Verification items for the finished model (mm, model axes). Give positions to 0.01 mm unless a question says otherwise; leave off trailing zeros. Write each loop counter-clockwise with the first axis right and the second up, starting at its lowest first coordinate (ties: lowest second). Pieces come first, ordered by that corner, then holes. Notation, with made-up numbers: (1, 68) -> (56, 68) arc R25 ccw to (56, 98) -> close; hole circle Ø5 at (3.5, -26.5). An arc over 180 degrees is marked (long way). Write item = value, one per line.
from build123d import *

# Parameters (mm, degrees)
SKETCH1_R           = 12.5
SKETCH1_R_2         = 1.5
SKETCH1_R_3         = 6
SKETCH1_R_4         = 4
BOSS_EXTRUDE1_DEPTH = 3
BOSS_EXTRUDE2_START = 3
SKETCH1_3_R         = 6
SKETCH1_3_R_2       = 4
BOSS_EXTRUDE2_DEPTH = 10


with BuildPart() as part:
    # Sketch1 → Boss-Extrude1 (new body)
    # profile 1 of 2: a face of its own
    with BuildSketch(Plane(origin=(0, 0, 0), x_dir=(1, 0, 0), z_dir=(0, 1, 0))):
        with Locations(Location((0, 0, 0), (0, 0, 270))):
            Circle(SKETCH1_R)
        with Locations(Location((-10, 0, 0), (0, 0, 270))):
            Circle(SKETCH1_R_2, mode=Mode.SUBTRACT)
        with Locations(Location((0, -10, 0), (0, 0, 270))):
            Circle(SKETCH1_R_2, mode=Mode.SUBTRACT)
        with Locations(Location((10, 0, 0), (0, 0, 270))):
            Circle(SKETCH1_R_2, mode=Mode.SUBTRACT)
        with Locations(Location((0, 10, 0), (0, 0, 270))):
            Circle(SKETCH1_R_2, mode=Mode.SUBTRACT)
        Circle(SKETCH1_R_3, mode=Mode.SUBTRACT)
    # profile 2 of 2: a face of its own
    with BuildSketch(Plane(origin=(0, 0, 0), x_dir=(1, 0, 0), z_dir=(0, 1, 0))):
        Circle(SKETCH1_R_3)
        with Locations(Location((0, 0, 0), (0, 0, 270))):
            Circle(SKETCH1_R_4, mode=Mode.SUBTRACT)
    extrude(amount=BOSS_EXTRUDE1_DEPTH)

    # Sketch1_3 → Boss-Extrude2 (add)
    with BuildSketch(Plane(origin=(0, 0, 0), x_dir=(1, 0, 0), z_dir=(0, 1, 0)).offset(BOSS_EXTRUDE2_START)):
        with Locations(Location((0, 0, 0), (0, 0, 270))):
            Circle(SKETCH1_3_R)
        with Locations(Location((0, 0, 0), (0, 0, 270))):
            Circle(SKETCH1_3_R_2, mode=Mode.SUBTRACT)
    extrude(amount=BOSS_EXTRUDE2_DEPTH)


solid = part.part
Item 1: Mould release check, pull along X, two halves, no side actions. Record for faces 1 (the cylindrical face through (0.07, 1.48, 8.5)), 2 (the flat face through (5.4, 3, -3)), 3 (the cylindrical face through (1.802, 7.93, 5.723)): +X half, -X half, draft (parallel to the pull), parting line (faces both ways), or undercut.
Response values:
face_1 = undercut
face_2 = draft
face_3 = parting line
Item 2: Sectioned sample at C-C on x = 0. Record the cut outline in (y, z), then the cut area to 3 significant figures.
Response values:
outline = (0, -12.5) -> (3, -12.5) -> (3, -11.5) -> (0, -11.5) -> close; (0, -8.5) -> (3, -8.5) -> (3, -6) -> (13, -6) -> (13, -4) -> (0, -4) -> close; (0, 4) -> (13, 4) -> (13, 6) -> (3, 6) -> (3, 8.5) -> (0, 8.5) -> close; (0, 11.5) -> (3, 11.5) -> (3, 12.5) -> (0, 12.5) -> close
area = 73.0 mm^2
Item 3: Go/stop test with flat-tipped pins: P1, Ø1, axis at y = 5, z = 7.5, coming from the +X side; P2, Ø6, axis at x = -6.5, y = 5.5, coming from the -Z side; P3, Ø1.5, axis at y = 5, z = -3, coming from the -X side; P4, Ø3.5, axis at x = 0, z = 10, coming from the +Y side. Record where each tip stops, or that it passes through.
Response values:
P1 = through
P2 = -11.52
P3 = -5.56
P4 = 3
Item 4: Sectioned sample at A-A on x = -10. Record the cut outline in (y, z), then the cut area to 3 significant figures.
Response values:
outline = (0, -7.5) -> (3, -7.5) -> (3, -1.5) -> (0, -1.5) -> close; (0, 1.5) -> (3, 1.5) -> (3, 7.5) -> (0, 7.5) -> close
area = 36.0 mm^2
Item 5: Material ranges on line 1 (X direction, y = 2.1, z = 0); line 2 (X direction, y = 4.25, z = -3.25); line 3 (X direction, y = 1.9, z = 10), recorded low to high.
Response values:
line_1 = -12.5 to -11.5, -8.5 to -4, 4 to 8.5, 11.5 to 12.5
line_2 = -5.04 to -2.33, 2.33 to 5.04
line_3 = -7.5 to -1.5, 1.5 to 7.5
Item 6: Sectioned sample at B-B on z = 0. Record the cut outline in (x, y).
Response values:
outline = (-12.5, 0) -> (-11.5, 0) -> (-11.5, 3) -> (-12.5, 3) -> close; (-8.5, 0) -> (-4, 0) -> (-4, 13) -> (-6, 13) -> (-6, 3) -> (-8.5, 3) -> close; (4, 0) -> (8.5, 0) -> (8.5, 3) -> (6, 3) -> (6, 13) -> (4, 13) -> close; (11.5, 0) -> (12.5, 0) -> (12.5, 3) -> (11.5, 3) -> close
Item 7: Sectioned sample at D-D on y = 1. Record the cut outline in (x, z).
Response values:
outline = circle Ø25 at (0, 0); hole circle Ø3 at (-10, 0); hole circle Ø8 at (0, 0); hole circle Ø3 at (0, -10); hole circle Ø3 at (0, 10); hole circle Ø3 at (10, 0)
